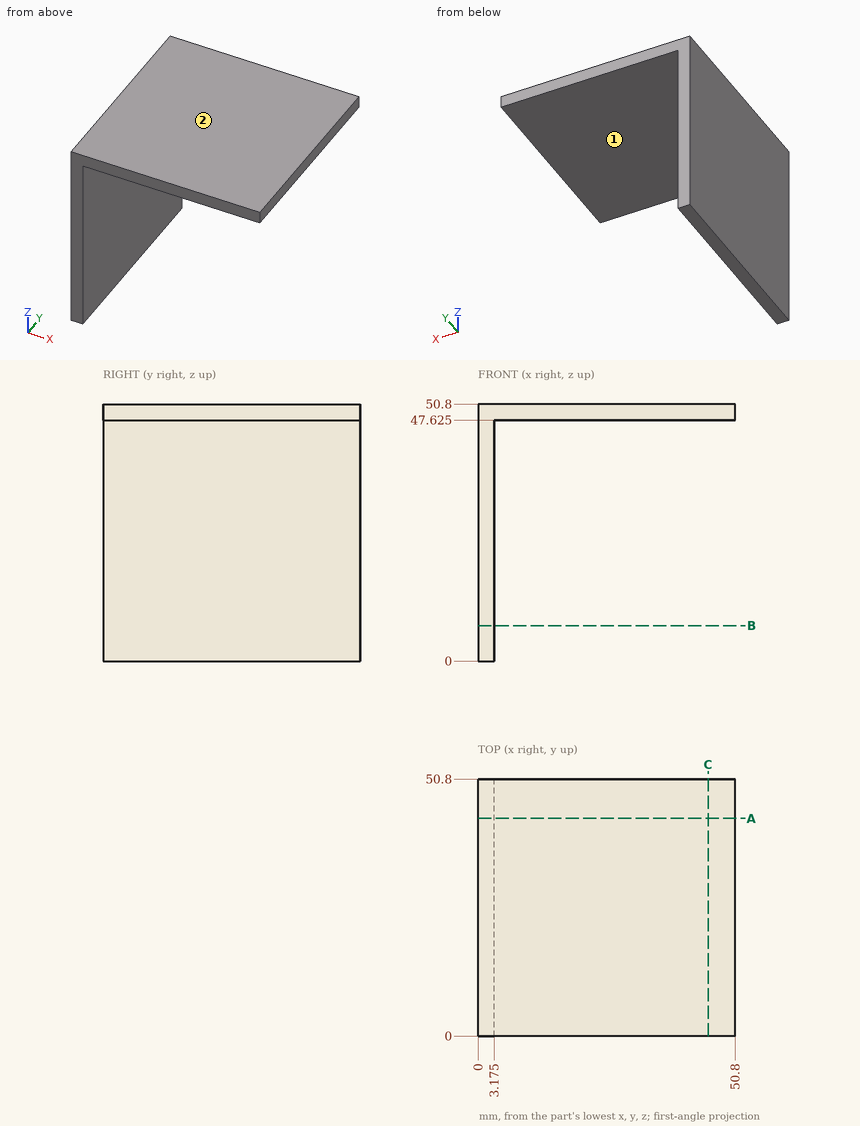
Could you check a few things on this drawing? It's one solid part, dimensions in mm from its lowest x, y, z. A direction names the side the tool comes from. Coordinates: 2 decimals unless noted, no trailing zeros. Order: outer loops, then holes, each group sorted by start corner. A loop starts at its lowest first (then second) coordinate and runs counter-clockwise, first axis right, second up. Notation, with made-up numbers: M 40.5,12 L 83.5,12 A13 cw 83.5,23 Z; hole C -30.75,9.5 d2. An arc over 180 degrees is marked long. Use one line per item in the form item = value. Start each with the question number.
1. Suppose I cut it at B-B on z = 7. Write out the boundary of the cut face in (x, y) (3 decimals), then the cut area to 3 significant figures.
2. For pin 1 (1.5 mm diameter, centred on x = 34.5, y = 34.5, fed in from -Z) (3 decimals); pin 2 (2 mm diameter, centred on y = 42, z = 10, fed in from +X) (3 decimals), each with a flat end and sliding along its axis, tell me the tip position at first contact or that it passes through.
3. Suppose I cut it at A-A on y = 43. Write out the boundary of the cut face in (x, z) (3 decimals), then the cut area to 4 significant figures.
4. Suppose I cut it at C-C on x = 45.5. Write out the boundary of the cut face in (y, z) (3 decimals), then the cut area to 3 significant figures.
5. On a 3-axis mill with a long thin cutter (end or side, diameter ignored), from which of +Z, -Z, +X, -X, +Y, -Y can I reach the whole of each face in a straight line? I mean the marked faces 1 and 2. Say none if no direction works.
6. Please list where these lines run through material, in increasing order: line 1 (Z direction, x = 15, y = 15) (3 decimals); line 2 (X direction, y = 19.5, z = 18.5) (3 decimals).
Geometry says:
q1.outline = M 0,0 L 3.175,0 L 3.175,50.8 L 0,50.8 Z
q1.area = 161 mm^2
q2.pin_1 = 47.625
q2.pin_2 = 3.175
q3.outline = M 0,0 L 3.175,0 L 3.175,47.625 L 50.8,47.625 L 50.8,50.8 L 0,50.8 Z
q3.area = 312.5 mm^2
q4.outline = M 0,47.625 L 50.8,47.625 L 50.8,50.8 L 0,50.8 Z
q4.area = 161 mm^2
q5.face_1 = -Z, +X, +Y, -Y
q5.face_2 = +Z, +X, -X, +Y, -Y
q6.line_1 = 47.625 to 50.8
q6.line_2 = 0 to 3.175
